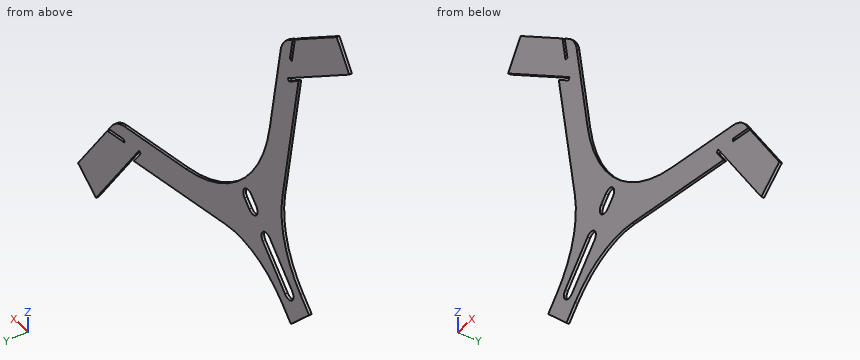
```python
from build123d import *

# Parameters (mm, degrees)
F1_DEPTH = 3.429


# Not quite as in the source:
# - ends of sketch curves that miss each other by under 0.0002 mm in the source are joined


with BuildPart() as f1:
    # F0 (on Front) → F1 (new body)
    with BuildSketch(Plane.XZ):
        with BuildLine():
            Line((-198.875523, -331.3710416), (-198.2139038, -327.6189282))
            Line((-198.2139038, -327.6189282), (-168.4471104, -332.867635))
            Line((-168.4471104, -332.867635), (-174.023655, -324.9035158))
            ThreePointArc((-174.023655, -324.9035158), (-184.7622274276, -314.6235496681), (-198.6173544615, -309.2355853348))
            Line((-198.6173544615, -309.2355853348), (-319.9769826, -287.83661))
            ThreePointArc((-319.9769826, -287.83661), (-428.3757561371, -231.4077731371), (-484.8045910801, -123.0089992615))
            Line((-484.8045910801, -123.0089992615), (-506.203585, -1.649349))
            ThreePointArc((-506.203585, -1.649349), (-511.5915580136, 12.2057554868), (-521.8715008941, 22.9443250094))
            Line((-521.8715008941, 22.9443250094), (-529.835618, 28.5208726))
            Line((-529.835618, 28.5208726), (-524.5869112, -1.2459208))
            Line((-524.5869112, -1.2459208), (-528.33905, -1.9075146))
            Line((-528.33905, -1.9075146), (-534.2493252, 31.6113922))
            Line((-534.2493252, 31.6113922), (-616.5409056, 89.2325622))
            Line((-616.5409056, 89.2325622), (-641.3079376, 53.861589))
            Line((-641.3079376, 53.861589), (-520.4086366, -30.7930042))
            Line((-520.4086366, -30.7930042), (-522.5939764, -33.9139784))
            Line((-522.5939764, -33.9139784), (-541.541589, -20.6467202))
            Line((-541.541589, -20.6467202), (-509.8508218, -200.3739452))
            ThreePointArc((-509.8508218, -200.3739452), (-513.7993593908, -260.6169022992), (-545.1188511893, -312.2298278107))
            Line((-545.1188511893, -312.2298278107), (-562.3549332, -329.4659146))
            Line((-562.3549332, -329.4659146), (-526.4338976, -365.3869248))
            Line((-526.4338976, -365.3869248), (-509.1978386, -348.1508658))
            ThreePointArc((-509.1978386, -348.1508658), (-457.5849106992, -316.8313763908), (-397.341954706, -312.8828450725))
            Line((-397.341954706, -312.8828450725), (-217.6147032, -344.573606))
            Line((-217.6147032, -344.573606), (-230.8819614, -325.6259934))
            Line((-230.8819614, -325.6259934), (-227.7609872, -323.4406536))
            Line((-227.7609872, -323.4406536), (-143.106394, -444.3399292))
            Line((-143.106394, -444.3399292), (-107.7354208, -419.5728972))
            Line((-107.7354208, -419.5728972), (-165.3565908, -337.2813422))
            Line((-165.3565908, -337.2813422), (-198.875523, -331.3710416))
        make_face()
        with BuildLine():
            ThreePointArc((-484.9002250908, -274.4618325092), (-471.4298472592, -274.4618261592), (-471.4298282092, -287.9322039908))
            Line((-471.4298282092, -287.9322039908), (-515.2085708, -331.7109698))
            ThreePointArc((-515.2085708, -331.7109698), (-528.6789538908, -331.7109708908), (-528.6789538908, -318.2405867092))
            Line((-528.6789538908, -318.2405867092), (-484.9002250908, -274.4618325092))
        make_face(mode=Mode.SUBTRACT)
        with BuildLine():
            ThreePointArc((-448.9791894908, -238.5408223092), (-435.5088053092, -238.5408223092), (-435.5088053092, -252.0112064908))
            Line((-435.5088053092, -252.0112064908), (-444.4890526, -260.9914516))
            ThreePointArc((-444.4890526, -260.9914516), (-457.9594356908, -260.9914526908), (-457.9594356908, -247.5210685092))
            Line((-457.9594356908, -247.5210685092), (-448.9791894908, -238.5408223092))
        make_face(mode=Mode.SUBTRACT)
    extrude(amount=F1_DEPTH)


solid = f1.part
```
Geometry: final body of the model. Coordinates: model frame, mm. Coordinates: 2 decimals unless noted, no trailing zeros. Order: outer loops, then holes, each group sorted by start corner. A loop starts at its lowest first (then second) coordinate and runs counter-clockwise, first axis right, second up.
Item 1: Section query A-A (z = -281). Output: boundary loops of the cut face in (x, y).
Answer:
outline: (-522.23, -3.43) - (-491.44, -3.43) - (-491.44, 0) - (-522.23, 0) - close; (-468.64, -3.43) - (-347.42, -3.43) - (-347.42, 0) - (-468.64, 0) - close
Item 2: Section query C-C (x = -408). Output: boundary loops of the cut face in (y, z), then the cut area to 3 significant figures.
Answer:
outline: (-3.43, -311.47) - (0, -311.47) - (0, -249.23) - (-3.43, -249.23) - close
area: 213 mm2
Item 3: Section query D-D (z = -177). Output: boundary loops of the cut face in (x, y), then the cut area to 3 significant figures.
Answer:
outline: (-513.97, -3.43) - (-467.23, -3.43) - (-467.23, 0) - (-513.97, 0) - close
area: 160 mm2
Item 4: Material intervals for line 1 along Z through (x, y) = (-447, -0.4); line 2 along X through (y, z) = (-0.2, -422); line 3 along Z through (x, y) = (-167, -0.55), sorted ascending.
Answer:
line 1: z = -313.99 to -262.79, -237.02 to -209.98
line 2: x = -158.75 to -111.2
line 3: z = -410.22 to -336.99
Item 5: Contact query for flat-ended pins moving along their axis: P1, Ø2, axis at y = -2, z = -135, coming from the -X side; P2, Ø1.5, axis at x = -502.5, y = -2, coming from the -Z side. Output: stop coordinate, or through.
Answer:
P1: stops at x = -521.55
P2: stops at z = -342.57
Item 6: Section query B-B (y = -2.6). State how many separate pieces and enclosed holes the cut face has, then the cut area to 3 significant figures.
Answer:
separate pieces: 1
enclosed holes: 2
area: 39,100 mm2
